from build123d import *

# Parameters (mm, degrees)
BOSS_EXTRUDE1_DEPTH        = 25.4
SKETCH13_W                 = 4.4958
SKETCH13_H                 = 17.78
CUT_EXTRUDE2_DEPTH         = 41.37401709
CONVERT_SOLID1_DEPTH       = 6.35
CONVERT_SOLID1_2_DEPTH     = 2.032
CONVERT_SOLID1_START       = 2.032
CONVERT_SOLID1_3_OUTLINE_W = 5.842
CONVERT_SOLID1_3_OUTLINE_H = 0.9144
CONVERT_SOLID1_3_DEPTH     = 4.318
CONVERT_SOLID1_START_2     = -0.9144
CONVERT_SOLID1_4_DEPTH     = 0.9144
CHAMFER1_SIZE              = 0.508
CUT_EXTRUDE3_DEPTH         = 32.703524625


with BuildPart() as part:
    # Sketch3 → Boss-Extrude1 (new body)
    with BuildSketch(Plane.XY):
        Polygon((6.35, 24.892), (6.35, 30.734), (0, 30.734), (0, 0), (2.032, 0), (2.032, 22.194824253), (4.064, 23.368), (4.064, 24.892), align=None)
    extrude(amount=BOSS_EXTRUDE1_DEPTH)

    # Sketch13 → Cut-Extrude2 (cut, through all)
    with BuildSketch(Plane(origin=(0, 0, 0), x_dir=(0, 0, -1), z_dir=(1, 0, 0))):
        with Locations((-2.2479, 8.89)):
            Rectangle(SKETCH13_W, SKETCH13_H)
    extrude(amount=CUT_EXTRUDE2_DEPTH, mode=Mode.SUBTRACT)

    # Convert-Solid1: read off the stored shape, not the designer's step
    # Convert-Solid1 outline → Convert-Solid1 (cut)
    with BuildSketch(Plane.YZ):
        with BuildLine():
            Line((30.734, 0), (30.734, 25.4))
            Line((30.734, 25.4), (0, 25.4))
            Line((0, 25.4), (0, 4.4958))
            Line((0, 4.4958), (17.78, 4.4958))
            Line((17.78, 4.4958), (17.78, 0.762))
            ThreePointArc((17.78, 0.762), (18.003184633, 0.223184633), (18.542, 0))
            Line((18.542, 0), (30.734, 0))
        make_face()
    extrude(amount=CONVERT_SOLID1_DEPTH, mode=Mode.SUBTRACT)

    # Convert-Solid1 2 outline → Convert-Solid1 2 (add)
    with BuildSketch(Plane.YZ):
        with BuildLine():
            Line((30.734, -0.9144), (30.734, 0))
            Line((30.734, 0), (17.78, 0))
            Line((17.78, 0), (17.78, 2.8194))
            ThreePointArc((17.78, 2.8194), (17.288993808, 4.004793808), (16.1036, 4.4958))
            Line((16.1036, 4.4958), (0, 4.4958))
            Line((0, 4.4958), (0, 3.5814))
            Line((0, 3.5814), (16.1036, 3.5814))
            ThreePointArc((16.1036, 3.5814), (16.642415367, 3.358215367), (16.8656, 2.8194))
            Line((16.8656, 2.8194), (16.8656, 0.762))
            ThreePointArc((16.8656, 0.762), (17.356606192, -0.423393808), (18.542, -0.9144))
            Line((18.542, -0.9144), (30.734, -0.9144))
        make_face()
    extrude(amount=CONVERT_SOLID1_2_DEPTH)

    # Convert-Solid1 3 outline → Convert-Solid1 3 (add)
    with BuildSketch(Plane.YZ.offset(CONVERT_SOLID1_START)):
        with Locations((27.813, -0.4572)):
            Rectangle(CONVERT_SOLID1_3_OUTLINE_W, CONVERT_SOLID1_3_OUTLINE_H)
    extrude(amount=CONVERT_SOLID1_3_DEPTH)

    # Convert-Solid1 4 outline → Convert-Solid1 4 (add)
    with BuildSketch(Plane.XY.offset(CONVERT_SOLID1_START_2)):
        Polygon((4.064, 23.368), (4.064, 24.892), (2.032, 24.892), (2.032, 22.194824253), align=None)
    extrude(amount=CONVERT_SOLID1_4_DEPTH)

    # Chamfer1
    chamfer1_edges = [part.edges().sort_by_distance(p)[0] for p in [
        (6.35, 24.892, -0.4572),
        (6.35, 30.734, -0.4572),
    ]]
    chamfer(chamfer1_edges, length=CHAMFER1_SIZE)

    # Sketch14 → Cut-Extrude3 (cut, through all)
    with BuildSketch(Plane.XY):
        Polygon((5.08, 16.129), (1.651, 12.7), (5.08, 9.271), align=None)
        Polygon((1.651, 0), (5.08, 3.429), (5.08, -3.429), align=None)
    extrude(amount=CUT_EXTRUDE3_DEPTH, mode=Mode.SUBTRACT)

    # Mirror1: part across plane


with BuildPart() as part_1:
    add(part.part)
    add(part.part.mirror(Plane(origin=(0, 0, 0), x_dir=(0, 0, 1), z_dir=(1, 0, 0))))

    # Mirror2: part across face


with BuildPart() as part_2:
    add(part_1.part)
    add(part_1.part.mirror(Plane(origin=(0, 0, 4.0386), x_dir=(0, 0, 1), z_dir=(0, -1, 0))))


solid = part_2.part
Check sheet for the modelled part. Datum: model origin and axes. Units: mm. A direction names the side the tool comes from. Give positions to 0.01 mm unless a question says otherwise; leave off trailing zeros. Loops run counter-clockwise (first coordinate to the right, second up) from the corner with the lowest first, then second, coordinate; pieces in that order, holes last. Notation, with made-up numbers: M -37,54 L -12,54 A22 cw -12,75 Z; hole C 63.25,35.5 d1. An arc over 180 degrees is marked long. Use a Markdown table: item, result. Add a question column.
Q1. Sectioned sample at D-D, the plane x = -3. Record the cut outline in (y, z), then the cut area to 3 significant figures.
Q2. Mould release check, pull along Y, two halves, no side actions. Record for faces 1 (the flat face through (0, 0, 4.496)), 2 (the cylindrical face through (0.028, -17.302, 3.992)), 3 (the flat face through (2.032, -17.6, 1.6)): pulls with the +Y half, pulls with the -Y half, needs draft (parallel to the pull), parting line crosses it, or undercut.
Q3. Tool access check on faces 4 (the flat face through (3.03, -22.77, -0.46)), 5 (the flat face through (0, -26, 0)), 6 (the flat face through (-2.032, -17.6, 1.6)), 7 (the cylindrical face through (0.028, 17.344, -0.41)). Record the directions out of +Z, -Z, +X, -X, +Y, -Y that give a thin tool (end or side, any length) a straight path to the whole face; none if there is none.
Q4. Scan lines: line 1 along Y through (x, z) = (-5.25, -0.55); line 2 along Z through (x, y) = (-0.5, -20); line 3 along Y through (x, z) = (0.75, 2.6). Record each from-to range of solid material in increasing order. Write a range as [from, to].
Q5. Sectioned sample at C-C, the plane y = 15.5. Record the cut outline in (x, z).
Q6. Sectioned sample at B-B, the plane x = 0.75. Record the cut outline in (y, z), then the cut area to 3 significant figures.
Q7. Sectioned sample at A-A, the plane x = -5.25. Record the cut outline in (y, z).
Q8. Go/stop test with flat-tipped pins: pin 1 (1 mm diameter, centred on x = 0.5, z = 2, fed in from -Y); pin 2 (0.7 mm diameter, centred on y = -4.5, z = 4, fed in from -X); pin 3 (4 mm diameter, centred on x = -0.5, y = -3, fed in from -Z); pin 4 (1.5 mm diameter, centred on x = -4.5, y = -1, fed in from +Z). Record where each tip stops, or that it passes through.
Verdict:
| question | item | result |
|---|---|---|
| 1 | outline | M -30.73,-0.91 L -22.75,-0.91 L -22.75,0 L -30.73,0 Z; M 22.75,-0.91 L 30.73,-0.91 L 30.73,0 L 22.75,0 Z |
| 1 | area | 14.6 mm^2 |
| 2 | face 1 | needs draft |
| 2 | face 2 | pulls with the -Y half |
| 2 | face 3 | undercut |
| 3 | face 4 | +Z, -Z, +X |
| 3 | face 5 | +Z, +X, -X, -Y |
| 3 | face 6 | +Z, -Z, -X |
| 3 | face 7 | -Z, +X, -X |
| 4 | line 1 | [-30.73, -24.89], [24.89, 30.73] |
| 4 | line 2 | [-0.91, 0] |
| 4 | line 3 | [-17.78, -16.87], [16.87, 17.78] |
| 5 | outline | M -2.03,3.58 L 2.03,3.58 L 2.03,4.5 L -2.03,4.5 Z |
| 6 | outline | M -30.73,-0.91 L -18.54,-0.91 A1.68 ccw -16.87,0.76 L -16.87,2.82 A0.76 cw -16.1,3.58 L 16.1,3.58 A0.76 cw 16.87,2.82 L 16.87,0.76 A1.68 ccw 18.54,-0.91 L 30.73,-0.91 L 30.73,0 L 18.54,0 A0.76 cw 17.78,0.76 L 17.78,2.82 A1.68 ccw 16.1,4.5 L -16.1,4.5 A1.68 ccw -17.78,2.82 L -17.78,0.76 A0.76 cw -18.54,0 L -30.73,0 Z |
| 6 | area | 62.5 mm^2 |
| 7 | outline | M -30.73,-0.91 L -24.89,-0.91 L -24.89,0 L -30.73,0 Z; M 24.89,-0.91 L 30.73,-0.91 L 30.73,0 L 24.89,0 Z |
| 8 | pin 1 | y = -17.78 |
| 8 | pin 2 | x = -2.03 |
| 8 | pin 3 | z = 3.58 |
| 8 | pin 4 | through |
